Build history of the part. All positions in model axes, mm. Round coordinates to 2 decimals unless told otherwise and drop trailing zeros. Order: outer loops, then holes, each group sorted by start corner. A loop starts at its lowest first (then second) coordinate and runs counter-clockwise, first axis right, second up. Notation, with made-up numbers: M 52,2 L 76,2 A23 ccw 76,39 Z; hole C 18,-5.5 d1. An arc over 180 degrees is marked long. One line per item, written item: value. Start each with the question number.
Item 1: Pin check, flat tips, straight feed: pin 1 (1 mm diameter, centred on x = 5, z = 24.5, fed in from -Y); pin 2 (0.6 mm diameter, centred on y = -10, z = 24, fed in from +X); pin 3 (3 mm diameter, centred on x = -12.35, y = -38.05, fed in from -Z); pin 4 (0.6 mm diameter, centred on y = -11, z = 23.5, fed in from -X). Stop position of each tip, or through.
Item 2: Band-saw the part on C-C, the plane z = 24. Write the cut outline in (x, y), then the cut area to 3 significant figures.
Item 3: Two-plate mould, pull along X, no slides. Class faces 1 (the cylindrical face through (-10.3, -46.37, 23.99)), 2 (the cylindrical face through (-38.383, -0.67, 24.014)), 3 (the flat face through (-1, 1, 23)): +X half, -X half, draft (parallel to the pull), parting line (faces both ways), or undercut.
Item 4: Band-saw the part on A-A, the plane x = 0. Write the cut outline in (y, z).
Item 5: Band-saw the part on B-B, the plane y = 0. Write the cut outline in (x, z), then the cut area to 3 significant figures.
Item 6: Band-saw the part on D-D, the plane x = -40. Write the cut outline in (y, z).
Item 7: Probe L1, parallel to Y at x = 1, z = 23.95; L2, parallel to Y at x = 31.5, z = 24.65; L3, parallel to Y at x = -41.5, z = 23.65. List the from-to ranges inside material, lowest first.
```python
from build123d import *

# Parameters (mm, degrees)
SKETCH003_R     = 47.5
PAD001_DEPTH    = 2
SKETCH012_R     = 1.75
POCKET005_DEPTH = 5
SKETCH021_W     = 25
SKETCH021_H     = 3.5
SKETCH021_W_2   = 20
POCKET013_DEPTH = 5


with BuildPart() as part:
    # Sketch003 → Pad001 (new body)
    with BuildSketch(Plane.XY):
        Circle(SKETCH003_R)
    extrude(amount=PAD001_DEPTH)

    # Sketch012 (on Face3 of Pad001) → Pocket005 (cut)
    with BuildSketch(Plane.XY.offset(2)):
        with Locations((-12.363995, 38.041183)):
            Circle(SKETCH012_R)
        with Locations((-12.347418, -38.046567)):
            Circle(SKETCH012_R)
        with Locations((-40, 0)):
            Circle(SKETCH012_R)
        with Locations((32.356581, 23.51705)):
            Circle(SKETCH012_R)
        with Locations((32.366826, -23.502949)):
            Circle(SKETCH012_R)
    extrude(amount=-POCKET005_DEPTH, mode=Mode.SUBTRACT)

    # Sketch021 (on Face3 of Pocket005) → Pocket013 (cut)
    with BuildSketch(Plane.XY.offset(2)):
        with Locations((3.5, 10.25)):
            Rectangle(SKETCH021_W, SKETCH021_H)
        with Locations((6, -10.25)):
            Rectangle(SKETCH021_W_2, SKETCH021_H)
    extrude(amount=-POCKET013_DEPTH, mode=Mode.SUBTRACT)


with BuildPart() as part_1:
    # Body001 placement: moved
    add(part.part.moved(Location((0, 0, 23))))


solid = part_1.part
```
Output:
1. pin 1: stops at y = -47.29
1. pin 2: stops at x = 46.5
1. pin 3: passes through
1. pin 4: stops at x = -46.28
2. outline: C 0,0 d95; hole C -40,0 d3.5; hole C -12.36,38.04 d3.5; hole C -12.35,-38.05 d3.5; hole M -9,8.5 L 16,8.5 L 16,12 L -9,12 Z; hole M -4,-12 L 16,-12 L 16,-8.5 L -4,-8.5 Z; hole C 32.36,23.52 d3.5; hole C 32.37,-23.5 d3.5
2. area: 6,880 mm²
3. face 1: parting line
3. face 2: undercut
3. face 3: draft
4. outline: M -47.5,23 L -12,23 L -12,25 L -47.5,25 Z; M -8.5,23 L 8.5,23 L 8.5,25 L -8.5,25 Z; M 12,23 L 47.5,23 L 47.5,25 L 12,25 Z
5. outline: M -47.5,23 L -41.75,23 L -41.75,25 L -47.5,25 Z; M -38.25,23 L 47.5,23 L 47.5,25 L -38.25,25 Z
5. area: 183 mm²
6. outline: M -25.62,23 L -1.75,23 L -1.75,25 L -25.62,25 Z; M 1.75,23 L 25.62,23 L 25.62,25 L 1.75,25 Z
7. L1: y = -47.49 to -12, -8.5 to 8.5, 12 to 47.49
7. L2: y = -35.55 to -25.02, -21.98 to 21.99, 25.04 to 35.55
7. L3: y = -23.11 to -0.9, 0.9 to 23.11
